Part model, mm, in its own coordinate system. A direction names the side the tool comes from. Round coordinates to 2 decimals unless told otherwise and drop trailing zeros. Write each loop counter-clockwise with the first axis right and the second up, starting at its lowest first coordinate (ties: lowest second). Pieces come first, ordered by that corner, then holes. Notation, with made-up numbers: M -11.75,16.25 L 24.25,16.25 A19 ccw 24.25,35.25 Z; hole C 3,-14 d10. An arc over 180 degrees is marked long. One line per question, with ' | ' between items. Start each with the question number.
1) Saw through at D-D (x = 78). List the corners of the cut face in (y, z), plus the area to 3 significant figures.
2) Mould opens along X. For faces 4 (the face through (-107.95, -4, -10)), 5 (the face through (-1, -4, -33.338)), 6 (the face through (56.48, -5.67, 10.5)) say: pulls with the +X half, pulls with the -X half, needs draft (parallel to the pull), parting line crosses it, or undercut.
3) Tool access for faces 1 (the face through (105, -4, 0)), 2 (the face through (-105, -4, 0)), 3 (the face through (1, -4, 46.038)): list every direction of +Z, -Z, +X, -X, +Y, -Y with a clear straight run to the whole face (end or side of a thin tool).
4) Drop flat-ended pins along their axis: pin 1 Ø1 at (y, z) = (-2.5, 9) entering from -X; pin 2 Ø2.5 at (y, z) = (-2.5, 9.5) entering from +X; pin 3 Ø11.5 at (x, z) = (0, 6.35) entering from +Y; pin 4 Ø6 at (x, z) = (34.5, -6) entering from +Y. Give the stop position or say it passes through.
5) Saw through at A-A (x = 0). List the corners of the cut face in (y, z).
6) Saw through at B-B (y = -2). Give the number of separate pieces and of enclosed holes in the cut face, plus the area to 3 significant figures.
7) Wall check: probe 1 along Z at (x, y) = (0, -6.25); probe 2 along X at (y, z) = (-3.75, 1.5); probe 3 along Z at (x, y) = (59, -6). Give the ranges that are in metal, low to high. Write a range as [from, to].
8) Saw through at C-C (z = 29). List the corners of the cut face in (x, y).
```python
from build123d import *

# Parameters (mm, degrees)
F1_DEPTH       = 7.9375
F2_R           = 34.925
F3_R           = 12.7
F4_D           = 6.7564
F5_D           = 6.7564
F6_D           = 12.7
F7_R           = 7.9375
F8_D           = 7.9375
F8_CSINK_D     = 19.05
F8_CSINK_ANGLE = 86


with BuildPart() as f1:
    # F0 (on Front) → F1 (new body)
    with BuildSketch(Plane.XZ):
        Polygon((-107.95, 0), (-107.95, -33.3375), (107.95, -33.3375), (107.95, 0), (93.6625, 0), (93.6625, 46.0375), (-93.6625, 46.0375), (-93.6625, 0), align=None)
    extrude(amount=F1_DEPTH)

    # F2
    f2_edges = [f1.edges().sort_by_distance(p)[0] for p in [
        (-93.6625, -3.96875, 46.0375),
        (93.6625, -3.96875, 46.0375),
    ]]
    fillet(f2_edges, radius=F2_R)

    # F3
    f3_edges = [f1.edges().sort_by_distance(p)[0] for p in [
        (-107.95, -3.96875, -33.3375),
        (107.95, -3.96875, -33.3375),
    ]]
    fillet(f3_edges, radius=F3_R)

    # F4 (through all)
    with Locations(Plane(origin=(0, 0, 0), x_dir=(1, 0, 0), z_dir=(0, 1, 0))):
        with Locations((-101.6, 7.9375), (101.6, 7.9375)):
            Hole(F4_D / 2)

    # F5 (through all)
    with Locations(Plane(origin=(0, 0, 0), x_dir=(1, 0, 0), z_dir=(0, 1, 0))):
        with Locations((0, -20.6375)):
            Hole(F5_D / 2)

    # F6 (through all)
    with Locations(Plane(origin=(0, 0, 0), x_dir=(1, 0, 0), z_dir=(0, 1, 0))):
        with Locations((0, -6.35)):
            Hole(F6_D / 2)

    # F7
    f7_edges = [f1.edges().sort_by_distance(p)[0] for p in [
        (-93.6625, -3.96875, 0),
        (93.6625, -3.96875, 0),
    ]]
    fillet(f7_edges, radius=F7_R)

    # F8 (through all)
    with Locations(Plane(origin=(0, 0, 0), x_dir=(1, 0, 0), z_dir=(0, 1, 0))):
        with Locations((-55.5625, -6.3627), (55.5625, -6.3627)):
            CounterSinkHole(F8_D / 2, F8_CSINK_D / 2, counter_sink_angle=F8_CSINK_ANGLE)


solid = f1.part
```
Answer key:
1) outline: M -7.94,-33.34 L 0,-33.34 L 0,40.25 L -7.94,40.25 Z | area: 584 mm2
2) face 4: pulls with the -X half | face 5: needs draft | face 6: undercut
3) face 1: +Z, +X, +Y, -Y | face 2: +Z, -X, +Y, -Y | face 3: +Z, +X, -X, +Y, -Y
4) pin 1: stops at x = -93.66 | pin 2: stops at x = 93.66 | pin 3: passes through | pin 4: stops at y = 0
5) outline: M -7.94,-33.34 L 0,-33.34 L 0,0 L -7.94,0 Z; M -7.94,12.7 L 0,12.7 L 0,17.26 L -7.94,17.26 Z; M -7.94,24.02 L 0,24.02 L 0,46.04 L -7.94,46.04 Z
6) separate pieces: 1 | enclosed holes: 6 | area: 14,700 mm2
7) probe 1: z = [-33.34, 0], [12.7, 17.26], [24.02, 46.04] | probe 2: x = [-96.96, -59.13], [-52, -4.1], [4.1, 52], [59.13, 96.96] | probe 3: z = [-33.34, 4.38], [8.35, 46.04]
8) outline: M -88.73,-7.94 L 88.73,-7.94 L 88.73,0 L -88.73,0 Z
